from build123d import *

# Parameters (mm, degrees)
BOSS_EXTRUDE1_DEPTH = 45
CUT_EXTRUDE1_START  = -37
SKETCH3_R           = 13.864092281
CUT_EXTRUDE1_DEPTH  = 29
SKETCH4_R           = 5
CUT_EXTRUDE2_DEPTH  = 81.507898783


with BuildPart() as part:
    # Sketch1 → Boss-Extrude1 (new body)
    with BuildSketch(Plane.XY):
        with BuildLine():
            Line((0, 0), (-35.793601182, 15.486061941))
            Line((-35.793601182, 15.486061941), (-35.793601182, 42.486061941))
            Line((-35.793601182, 42.486061941), (-14.301302797, 42.486061941))
            ThreePointArc((-14.301302797, 42.486061941), (-0.437210516, 56.350154222), (13.426881764, 42.486061941))
            Line((13.426881764, 42.486061941), (34.919180149, 42.486061941))
            Line((34.919180149, 42.486061941), (34.919180149, 21.486061941))
            Line((34.919180149, 21.486061941), (0, 0))
        make_face()
    extrude(amount=BOSS_EXTRUDE1_DEPTH)

    # Sketch3 → Cut-Extrude1 (cut)
    with BuildSketch(Plane.XY.offset(45).offset(CUT_EXTRUDE1_START)):
        with Locations((-0.437210516, 42.486061941)):
            Circle(SKETCH3_R)
    extrude(amount=CUT_EXTRUDE1_DEPTH, mode=Mode.SUBTRACT)

    # Sketch4 → Cut-Extrude2 (cut, through all)
    with BuildSketch(Plane.XY.offset(45)):
        with Locations((-0.437210516, 42.486061941)):
            Circle(SKETCH4_R)
    extrude(amount=-CUT_EXTRUDE2_DEPTH, mode=Mode.SUBTRACT)


solid = part.part
Read the model definition and answer for the solid it produces. Units are mm, in the model's axes. A direction names the side the tool comes from. Round coordinates to 2 decimals unless told otherwise and drop trailing zeros. Loops run counter-clockwise (first coordinate to the right, second up) from the corner with the lowest first, then second, coordinate; pieces in that order, holes last.
Q1. Which of the six approach directions +Z, -Z, +X, -X, +Y, -Y give full straight-line access (tool end or side, diameter ignored) to faces 1 (the face through (-35.794, 29, 22)), 2 (the face through (24, 42.486, 22)), 3 (the face through (-25, 42.486, 22)), 4 (the face through (17.7, 10.89, 22.18)), 5 (the face through (6, 43, 8))?
Q2. Section A-A on z = 42 is taken. Write down the section's boundary in (x, y), and give its area (3 significant figures).
Q3. Section C-C on z = 17 is taken. Write down the section's boundary in (x, y).
Q4. Determine the mould class of faces 6 (the face through (0, 29, 0)), 7 (the face through (-0.742, 28.625, 22.297)), 8 (the face through (-1.5, 37.6, 4.1)), 9 (the face through (6, 43, 37)) for opening direction Z: released by +Z, released by -Z, zero draft, split by the parting line, or undercut.
Q5. Each of these flat-tipped pins is pushed along its axis until it touches: pin 1 (8 mm diameter, centred on x = -24, z = 6, fed in from -Y); pin 2 (1.5 mm diameter, centred on y = 14.5, z = 32, fed in from -X); pin 3 (17 mm diameter, centred on x = 21.5, z = 29.5, fed in from +Y). Where does it stop, or does it pass through?
Q6. Consider probe 1 along Z at (x, y) = (-0.5, 33); probe 2 along X at (y, z) = (39, 11.5); probe 3 along X at (y, z) = (31, 12). Determine where each line is inside the solid, lowest interval first.
Q7. Section B-B on y = 43.5 is taken. Write down the section's boundary in (x, z), and give its area (3 significant figures).
Q8. Section D-D on x = -3.5 is taken. Write down the section's boundary in (y, z), and give its area (3 significant figures).
Output:
1. face 1: +Z, -Z, -X, +Y, -Y
1. face 2: +Z, -Z, +X, +Y
1. face 3: +Z, -Z, -X, +Y
1. face 4: +Z, -Z, +X, -Y
1. face 5: +Y
2. outline: (-35.79, 15.49) - (0, 0) - (34.92, 21.49) - (34.92, 42.49) - (13.43, 42.49) arc R13.86 ccw to (-14.3, 42.49) - (-35.79, 42.49) - close; hole circle Ø10 at (-0.44, 42.49)
2. area: 2,580 mm2
3. outline: (-35.79, 15.49) - (0, 0) - (34.92, 21.49) - (34.92, 42.49) - (13.43, 42.49) arc R13.86 cw to (-14.3, 42.49) - (-35.79, 42.49) - close
4. face 6: released by -Z
4. face 7: undercut
4. face 8: zero draft
4. face 9: undercut
5. pin 1: stops at y = 8.65
5. pin 2: stops at x = -35.25
5. pin 3: stops at y = 42.49
6. probe 1: z = 0 to 8, 37 to 45
6. probe 2: x = -35.79 to -13.86, 12.98 to 34.92
6. probe 3: x = -35.79 to -8.2, 7.33 to 34.92
7. outline: (-14.26, 0) - (-5.33, 0) - (-5.33, 8) - (-14.26, 8) - close; (-14.26, 37) - (-5.33, 37) - (-5.33, 45) - (-14.26, 45) - close; (4.46, 0) - (13.39, 0) - (13.39, 8) - (4.46, 8) - close; (4.46, 37) - (13.39, 37) - (13.39, 45) - (4.46, 45) - close
7. area: 286 mm2
8. outline: (1.51, 0) - (38.53, 0) - (38.53, 8) - (28.96, 8) - (28.96, 37) - (38.53, 37) - (38.53, 45) - (1.51, 45) - close; (46.44, 0) - (56.01, 0) - (56.01, 8) - (46.44, 8) - close; (46.44, 37) - (56.01, 37) - (56.01, 45) - (46.44, 45) - close
8. area: 1,540 mm2
